For this review, take the finished solid that the model builds, in its own axes (mm). Face numbers are marked on the shaded views. A direction names the side the tool comes from. Give positions to 0.01 mm unless a question says otherwise; leave off trailing zeros. Loops run counter-clockwise (first coordinate to the right, second up) from the corner with the lowest first, then second, coordinate; pieces in that order, holes last.
```python
from build123d import *

# Parameters (mm, degrees)
F0_W     = 100
F0_H     = 80
F1_DEPTH = 5
F3_DEPTH = 100
F4_W     = 100
F4_H     = 5
F5_DEPTH = 30
F6_R     = 5
F7_DEPTH = 5
F8_W     = 100
F8_H     = 25
F9_DEPTH = 5


with BuildPart() as f1:
    # F0 (on Front) → F1 (new body)
    with BuildSketch(Plane.XZ):
        with Locations((26.364678, -15.465713)):
            Rectangle(F0_W, F0_H)
    extrude(amount=F1_DEPTH)

    # F2 (on face) → F3 (join)
    with BuildSketch(Plane.YZ.offset(76.364678)):
        with BuildLine():
            ThreePointArc((-25, 24.534287), (-10.857864, 18.676422), (-5, 4.534287))
            Line((-5, 4.534287), (-5, 24.534287))
            Line((-5, 24.534287), (-25, 24.534287))
        make_face()
        with BuildLine():
            ThreePointArc((-25, -15.465713), (-10.857864, -21.323578), (-5, -35.465713))
            Line((-5, -35.465713), (-5, 4.534287))
            ThreePointArc((-5, 4.534287), (-10.857864, -9.607849), (-25, -15.465713))
        make_face()
        with BuildLine():
            ThreePointArc((-5, -35.465713), (-10.857864, -49.607849), (-25, -55.465713))
            Line((-25, -55.465713), (-5, -55.465713))
            Line((-5, -55.465713), (-5, -35.465713))
        make_face()
    extrude(amount=-F3_DEPTH)

    # F4 (on face) → F5 (join)
    with BuildSketch(Plane(origin=(0, 0, -55.465713), x_dir=(1, 0, 0), z_dir=(0, 0, -1))):
        with Locations((26.364678, 2.5)):
            Rectangle(F4_W, F4_H)
    extrude(amount=F5_DEPTH)

    # F6 (on face) → F7 (cut)
    with BuildSketch(Plane.XZ.offset(5)):
        with Locations((66.364678, -75.465713)):
            Circle(F6_R)
        with Locations((-13.635322, -75.465713)):
            Circle(F6_R)
    extrude(amount=-F7_DEPTH, mode=Mode.SUBTRACT)

    # F8 (on face) → F9 (join)
    with BuildSketch(Plane.XY.offset(24.534287)):
        with Locations((26.364678, -12.5)):
            Rectangle(F8_W, F8_H)
    extrude(amount=F9_DEPTH)


solid = f1.part
```
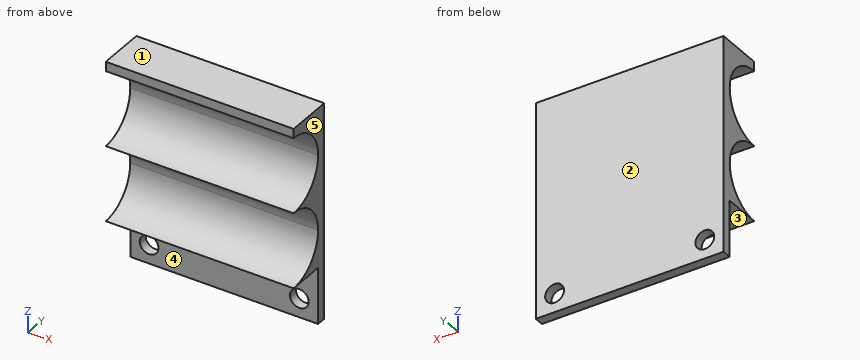
Item 1: Clearance check with flat-ended pins moving along their axes: pin 1 Ø1 at (x, z) = (5.5, 14.5) entering from +Y; pin 2 Ø6 at (x, y) = (-13.5, -20) entering from -Z; pin 3 Ø4 at (x, z) = (14, -34.5) entering from -Y; pin 4 Ø15 at (x, z) = (44.5, -65) entering from -Y. State where each tip first meets the part, or that it passes through.
Answer:
pin 1: stops at y = 0
pin 2: stops at z = -55.47
pin 3: stops at y = -5.22
pin 4: stops at y = -5
Item 2: Take a section at A-A on x = -12. Give the boundary of the cut face in (y, z).
Answer:
outline: (-25, -55.47) - (-5, -55.47) - (-5, -70.74) - (0, -70.74) - (0, 29.53) - (-25, 29.53) - (-25, 24.53) arc R20 cw to (-5, 4.53) arc R20 cw to (-25, -15.47) arc R20 cw to (-5, -35.47) arc R20 cw to start; (-5, -85.47) - (0, -85.47) - (0, -80.19) - (-5, -80.19) - close
Item 3: Take a section at C-C on z = -59. Give the boundary of the cut face in (x, y), and give its area (3 significant figures).
Answer:
outline: (-23.64, -5) - (76.36, -5) - (76.36, 0) - (-23.64, 0) - close
area: 500 mm2
Item 4: Take a section at B-B on y = -18.25. Give the boundary of the cut face in (x, z), and give its area (3 significant figures).
Answer:
outline: (-23.64, -55.47) - (76.36, -55.47) - (76.36, -54.29) - (-23.64, -54.29) - close; (-23.64, -16.64) - (76.36, -16.64) - (76.36, -14.29) - (-23.64, -14.29) - close; (-23.64, 23.36) - (76.36, 23.36) - (76.36, 29.53) - (-23.64, 29.53) - close
area: 969 mm2
Item 5: For L1, parallel to Z at x = -5, y = -13.75; L2, parallel to Z at x = 37, y = -20; L3, parallel to Y at x = 49.5, z = -74.5, list the stretches that pass through material, from the lowest coordinate up.
Answer:
L1: z = -55.47 to -52, -18.93 to -12, 21.07 to 29.53
L2: z = -55.47 to -54.83, -16.1 to -14.83, 23.9 to 29.53
L3: y = -5 to 0
Item 6: The part is to be moulded in two halves that separate along Z. For the marked faces 1, 2 and 3, say which applies: released by +Z, released by -Z, zero draft, split by the parting line, or undercut.
Answer:
face 1: released by +Z
face 2: zero draft
face 3: released by -Z
Item 7: Tool access review of the marked faces 4 and 5: name each direction out of +Z, -Z, +X, -X, +Y, -Y from which nothing blocks a thin tool from reaching the whole face with its end or side.
Answer:
face 4: -Z, +X, -X, -Y
face 5: +Z, -Z, +X, +Y, -Y
Item 8: Take a section at D-D on x = 5. Give the boundary of the cut face in (y, z), and give its area (3 significant figures).
Answer:
outline: (-25, -55.47) - (-5, -55.47) - (-5, -85.47) - (0, -85.47) - (0, 29.53) - (-25, 29.53) - (-25, 24.53) arc R20 cw to (-5, 4.53) arc R20 cw to (-25, -15.47) arc R20 cw to (-5, -35.47) arc R20 cw to start
area: 1,020 mm2
